from build123d import *

# Parameters (mm, degrees)
F0_W          = 20
F0_H          = 40
F1_DEPTH      = 4
F1_DEPTH_BACK = 4
F3_R          = 0.25
F6_R          = 0.25
F10_D         = 3
F10_DEPTH     = 11
F10_TIP       = 0.9012909285
F11_D         = 3
F11_DEPTH     = 11
F11_TIP       = 0.9012909285


with BuildPart() as f1:
    # F0 (on Top) → F1 (new body, two sides)
    with BuildSketch(Plane.XY) as f1_sk:
        Rectangle(F0_W, F0_H)
    extrude(amount=F1_DEPTH)
    extrude(f1_sk.sketch, amount=-F1_DEPTH_BACK)

    # F4: sweep along a path in F2
    with BuildLine(Plane.XY) as f4_path:
        Line((0, -20), (0, -5))
        Line((0, -5), (5, 2))
        Line((5, 2), (5, 20))
    # F3 (on face) → F4 (sweep, cut)
    with BuildSketch(Plane(origin=(0, 20, 0), x_dir=(-1, 0, 0), z_dir=(0, 1, 0))):
        with Locations((-5, 0)):
            Circle(F3_R)
    sweep(path=f4_path.line, transition=Transition.RIGHT, mode=Mode.SUBTRACT)

    # F7: sweep along a path in F5
    with BuildLine(Plane.XY) as f7_path:
        Line((0, -5), (-5, 2))
        Line((-5, 2), (-5, 20))
    # F6 (on face) → F7 (sweep, cut)
    with BuildSketch(Plane(origin=(0, 20, 0), x_dir=(-1, 0, 0), z_dir=(0, 1, 0))):
        with Locations((5, 0)):
            Circle(F6_R)
    sweep(path=f7_path.line, transition=Transition.RIGHT, mode=Mode.SUBTRACT)

    # F10
    with Locations(Plane(origin=(0, 20, 0), x_dir=(-1, 0, 0), z_dir=(0, 1, 0))):
        with Locations((-5, 0)):
            Hole(F10_D / 2, depth=F10_DEPTH)
            with Locations((0, 0, -(F10_DEPTH + F10_TIP / 2))):  # 118° drill point
                Cone(0, F10_D / 2, F10_TIP, mode=Mode.SUBTRACT)

    # F11
    with Locations(Plane(origin=(0, 20, 0), x_dir=(-1, 0, 0), z_dir=(0, 1, 0))):
        with Locations((5, 0)):
            Hole(F11_D / 2, depth=F11_DEPTH)
            with Locations((0, 0, -(F11_DEPTH + F11_TIP / 2))):  # 118° drill point
                Cone(0, F11_D / 2, F11_TIP, mode=Mode.SUBTRACT)


solid = f1.part
CAD build for the part. Positions are in the model's coordinates, mm. A direction names the side the tool comes from. Give positions to 0.01 mm unless a question says otherwise; leave off trailing zeros. Loops run counter-clockwise (first coordinate to the right, second up) from the corner with the lowest first, then second, coordinate; pieces in that order, holes last. Notation, with made-up numbers: M 82.5,14 L 137.5,14 A20 cw 137.5,26 Z; hole C 32,21 d2. An arc over 180 degrees is marked long. One line per question, with ' | ' between items. Start each with the question number.
1. Two-plate mould, pull along Y, no slides. Class faces 1 (the face through (-6.2, 14.4, -0.9)), 2 (the face through (-2.747, -1.552, -0.096)), 3 (the face through (0, 20, 0)): pulls with the +Y half, pulls with the -Y half, needs draft (parallel to the pull), parting line crosses it, or undercut.
2. Probe L1, parallel to Z at x = 5, y = 17.5; L2, parallel to Z at x = -5, y = 7.25; L3, parallel to X at y = 3.5, z = 0. List the from-to ranges inside material, lowest first. Write a range as from..to.
3. 3-axis set-ups, long thin cutter, end or side, ignore diameter. For faces 4 (the face through (-10, 0, 0)), 5 (the face through (6.386, 14.423, -0.575)): which of +Z, -Z, +X, -X, +Y, -Y reach the whole face in a straight line?
4. Saw through at A-A on y = 17. Give the cut face in (x, z), plus the area to 3 significant figures.
Result sheet:
1) face 1: needs draft | face 2: undercut | face 3: pulls with the +Y half
2) L1: z = -4..-1.5, 1.5..4 | L2: z = -4..-0.25, 0.25..4 | L3: x = -10..-5.25, -4.75..4.75, 5.25..10
3) face 4: +Z, -Z, -X, +Y, -Y | face 5: +Y
4) outline: M -10,-4 L 10,-4 L 10,4 L -10,4 Z; hole C -5,0 d3; hole C 5,0 d3 | area: 146 mm^2
